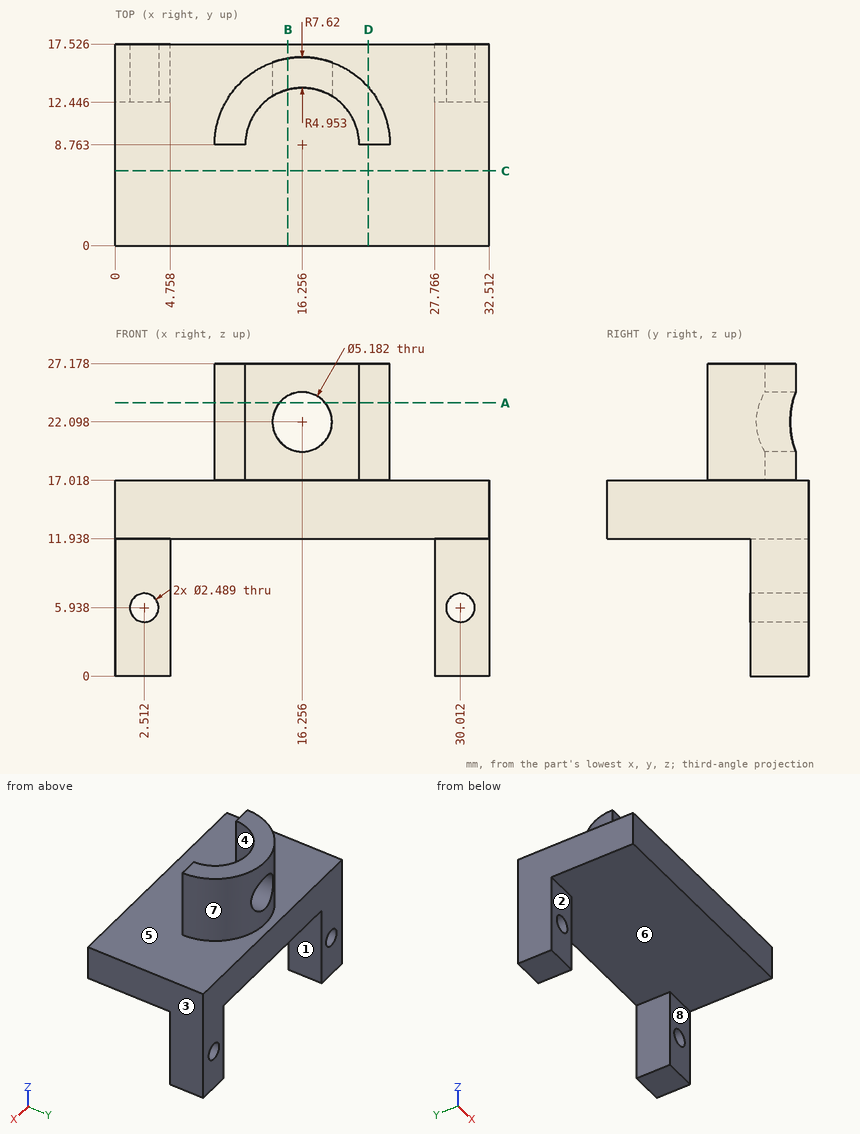
The drawing under review shows one solid part. Ordinate dimensions are in mm from its lowest x, y, z. A direction names the side the tool comes from. Coordinates: 2 decimals unless noted, no trailing zeros. Loops run counter-clockwise (first coordinate to the right, second up) from the corner with the lowest first, then second, coordinate; pieces in that order, holes last. Notation, with made-up numbers: (8.5, -31) -> (46.5, -31) arc R31 ccw to (46.5, 6) -> close; hole circle Ø10 at (27.25, 37). An arc over 180 degrees is marked (long way). Answer as a JSON object with one key per item and string values.
Q1. Take a section at D-D on x = 22. Give the boundary of the cut face in (y, z), plus the area to 3 significant figures.
Answer block:
{"outline": "(0, 11.94) -> (17.53, 11.94) -> (17.53, 17.02) -> (13.77, 17.02) -> (13.77, 27.18) -> (8.76, 27.18) -> (8.76, 17.02) -> (0, 17.02) -> close", "area": "140 mm^2"}
Q2. Take a section at B-B on x = 15. Give the boundary of the cut face in (y, z), plus the area to 3 significant figures.
Answer block:
{"outline": "(0, 11.94) -> (17.53, 11.94) -> (17.53, 17.02) -> (16.28, 17.02) -> (16.28, 19.83) -> (13.55, 19.83) -> (13.55, 17.02) -> (0, 17.02) -> close; (13.55, 24.36) -> (16.28, 24.36) -> (16.28, 27.18) -> (13.55, 27.18) -> close", "area": "104 mm^2"}
Q3. Take a section at C-C on y = 6.5. Give the boundary of the cut face in (x, z).
Answer block:
{"outline": "(0, 11.94) -> (32.51, 11.94) -> (32.51, 17.02) -> (0, 17.02) -> close"}
Q4. The part is to be moulded in two halves that separate along X. For the marked faces 6, 7 and 8, say which applies: +X half, -X half, draft (parallel to the pull), parting line (faces both ways), or undercut.
Answer block:
{"face 6": "undercut", "face 7": "parting line", "face 8": "draft"}
Q5. To check wall thickness, follow L1, parallel to X at y = 13, z = 6 (1 decimal); L2, parallel to X at y = 13, z = 9; L3, parallel to Y at x = 4, z = 11.5. State the ranges of each line that lie inside material, in increasing order.
Answer block:
{"L1": "x = 0 to 1.3, 3.8 to 4.8, 27.8 to 28.8, 31.3 to 32.5", "L2": "x = 0 to 4.76, 27.77 to 32.51", "L3": "y = 12.45 to 17.53"}
Q6. Tool access review of the marked faces 1, 2, 3, 4 and 5: name each direction out of +Z, -Z, +X, -X, +Y, -Y from which nothing blocks a thin tool from reaching the whole face with its end or side.
Answer block:
{"face 1": "-Z, +Y, -Y", "face 2": "-Z, +X, -X, -Y", "face 3": "+Z, -Z, +X, +Y, -Y", "face 4": "+Z, -Y", "face 5": "+Z"}
Q7. Clearance check with flat-ended pins moving along their axes: pin 1 Ø8 at (x, y) = (12, 4) entering from -Z; pin 2 Ø4 at (x, z) = (1.5, 3.5) entering from -Y; pin 3 Ø0.8 at (x, z) = (9.5, 22.5) entering from -Y; pin 4 Ø1.5 at (y, z) = (14, 8) entering from -X. State where each tip first meets the part, or that it passes through.
Answer block:
{"pin 1": "stops at z = 11.94", "pin 2": "stops at y = 12.45", "pin 3": "stops at y = 8.76", "pin 4": "stops at x = 0"}
Q8. Take a section at A-A on z = 23.75. Give the boundary of the cut face in (x, y).
Answer block:
{"outline": "(8.64, 8.76) -> (11.3, 8.76) arc R4.95 cw to (14.26, 13.3) -> (14.26, 16.12) arc R7.62 ccw to start; (18.25, 13.3) arc R4.95 cw to (21.21, 8.76) -> (23.88, 8.76) arc R7.62 ccw to (18.25, 16.12) -> close"}
